Part model, mm, in its own coordinate system. Face numbers are marked on the shaded views. A direction names the side the tool comes from. Coordinates: 2 decimals unless noted, no trailing zeros. Loops run counter-clockwise (first coordinate to the right, second up) from the corner with the lowest first, then second, coordinate; pieces in that order, holes last. Notation, with made-up numbers: (8.5, 51.5) - (44.5, 51.5) arc R14 cw to (44.5, 65.5) - close; hole circle Ø1 at (47.5, -17.5). An arc over 180 degrees is marked (long way). Use a Markdown table: item, result. Add a question column.
1) Pull direction X, two halves, no side cores. Call the marked faces 3 and 4: +X half, -X half, draft (parallel to the pull), parting line (faces both ways), or undercut.
2) Band-saw the part on A-A (x = 23). Give the cut face in (y, z).
3) Band-saw the part on D-D (x = 55). Give the cut face in (y, z), plus the area to 4 significant figures.
4) Drop flat-ended pins along their axis: P1, Ø5.5, axis at x = 23.5, z = 13.5, coming from the -Y side; P2, Ø2, axis at x = 42.5, y = 6, coming from the +Z side; P3, Ø8, axis at y = 44.5, z = 12, coming from the +X side. Give the stop position or say it passes through.
5) Band-saw the part on C-C (y = 95). Give the cut face in (x, z), plus the area to 3 significant figures.
6) Probe probe 1 along X at (y, z) = (143.8, 10.5); probe 2 along Y at (x, z) = (36.5, 8.75); probe 3 along X at (y, z) = (49, 28.75). List the from-to ranges inside material, lowest first. Write a range as [from, to].
7) Tool access for the marked faces 1 and 2: list every direction of +Z, -Z, +X, -X, +Y, -Y with a clear straight run to the whole face (end or side of a thin tool).
8) Band-saw the part on B-B (z = 4.75). Give the cut face in (x, y).
Autodesk Inventor part; units mm, degrees
ref_plane "Work Plane1" through (0, 0, 12.5) normal (0, 0, -1) x (-1, 0, 0)
ref_plane "YZ Plane" through (0, 0, 0) normal (1, 0, 0) x (0, 1, 0)
ref_plane "XZ Plane" through (0, 0, 0) normal (0, 1, 0) x (-1, 0, 0)
sketch "Sketch1" plane through (0, 0, 0) normal (0, 0, 1) x (1, 0, 0)
  line L0 (33.3378, 145.104) -> (83.3378, 145.104)
  line L1 (83.3378, 145.104) -> (83.3378, 5.104)
  line L2 (83.3378, 5.104) -> (33.3378, 5.104)
  line L3 (33.3378, 5.104) -> (33.3378, 145.104)
  line L4 (33.3378, 90.104) -> (33.3378, 60.104)
  line L5 (83.3378, 90.104) -> (83.3378, 60.104)
  point P0 (0, 0)
  dimension "d0" = 140
  dimension "d1" = 50
extrude "Extrusion1" add sketch "Sketch1" along normal blind 30
sketch "Sketch2" plane through (0, 0, 30) normal (0, 0, 1) x (1, 0, 0)
  line L0 (35.8378, 142.604) -> (80.8378, 142.604)
  line L1 (80.8378, 142.604) -> (80.8378, 7.604)
  line L2 (80.8378, 7.604) -> (35.8378, 7.604)
  line L3 (35.8378, 7.604) -> (35.8378, 142.604)
  line L4 (83.3378, 145.104) -> (33.3378, 145.104)
  line L5 (83.3378, 5.104) -> (83.3378, 145.104)
  line L6 (33.3378, 5.104) -> (83.3378, 5.104)
  line L7 (33.3378, 145.104) -> (33.3378, 5.104)
  point P0 (0, 0)
  point P1 (58.3378, 142.604)
  dimension "d4" = 2.5
  dimension "d5" = 2.5
  dimension "d6" = 2.5
  dimension "d7" = 2.5
extrude "Extrusion2" cut sketch "Sketch2" against normal blind 27 contours L0 L1 L2 L3
sketch "Sketch3" plane through (33.3378, 5.104, 0) normal (0, -1, 0) x (1, 0, 0)
  line L0 (7, 30) -> (37, 30)
  line L1 (37, 30) -> (37, 15)
  line L2 (37, 15) -> (7, 15)
  line L3 (7, 15) -> (7, 30)
  line L4 (0, 0) -> (50, 0)
  line L5 (0, 0) -> (0, 30)
  line L6 (0, 30) -> (50, 30)
  line L7 (10, 15) -> (35, 15)
  line L8 (35, 15) -> (35, 3)
  line L9 (35, 3) -> (10, 3)
  line L10 (10, 3) -> (10, 15)
  point P0 (-33.3378, 0)
  point P1 (37, 22.5)
  point P2 (10, 9)
  dimension "d10" = 15
  dimension "d11" = 30
  dimension "d12" = 7
  dimension "d13" = 0
  dimension "d14" = 25
  dimension "d15" = 10
  dimension "d16" = 3
extrude "Extrusion3" cut sketch "Sketch3" against normal blind 27
sketch "Sketch4" plane through (0, 0, 0) normal (0, 0, -1) x (-1, 0, 0)
  circle A0 centre (-74.8378, 13.604) radius 1.5
  circle A1 centre (-41.8378, 13.604) radius 1.5
  circle A2 centre (-41.8378, 99.604) radius 1.5
  circle A3 centre (-74.8378, 99.604) radius 1.5
  circle A4 centre (-41.8378, 111.604) radius 1.5
  circle A5 centre (-74.8378, 111.604) radius 1.5
  line L0 (-83.3378, 5.104) -> (-83.3378, 145.104)
  line L1 (-33.3378, 145.104) -> (-33.3378, 5.104)
  line L2 (-33.3378, 5.104) -> (-83.3378, 5.104)
  line L3 (-83.3378, 145.104) -> (-33.3378, 145.104)
  point P0 (0, 0)
  dimension "d19" = 8.5
  dimension "d20" = 8.5
  dimension "d21" = 8.5
  dimension "d22" = 8.5
  dimension "d23" = 3
  dimension "d24" = 3
  dimension "d25" = 8.5
  dimension "d26" = 8.5
  dimension "d27" = 8.5
  dimension "d28" = 8.5
  dimension "d29" = 3
  dimension "d30" = 3
  dimension "d31" = 3
  dimension "d32" = 3
  dimension "d33" = 12
  dimension "d34" = 12
  dimension "d35" = 33.5
  dimension "d36" = 33.5
extrude "Extrusion4" cut sketch "Sketch4" against normal blind 27 contours A0 | A1 | A2 | A3 | A4 | A5
sketch "Sketch5" plane through (33.3378, 145.104, 0) normal (0, 1, 0) x (1, 0, 0)
  circle A0 centre (35.5, -10.5) radius 2.5
  circle A1 centre (10.5, -10.5) radius 2.5
  line L0 (50, 0) -> (50, -30)
  line L1 (50, 0) -> (0, 0)
  point P0 (-33.3378, 0)
  dimension "d39" = 5
  dimension "d40" = 5
  dimension "d41" = 25
  dimension "d42" = 14.5
  dimension "d43" = 10.5
  dimension "d44" = 10.5
extrude "Extrusion5" cut sketch "Sketch5" against normal blind 27
sketch "Sketch6" plane through (33.3378, 5.104, 0) normal (0, -1, 0) x (1, 0, 0)
  point P0 (-33.3378, 0)
ref_plane "Work Plane1" through (0, 0, 12.5) normal (0, 0, -1) x (-1, 0, 0)
sketch "Sketch7" plane through (0, 0, 12.5) normal (0, 0, -1) x (-1, 0, 0)
  line L0 (-83.3378, 5.104) -> (-83.3378, 145.104)
  line L1 (-83.3378, 90.104) -> (-103.3378, 90.104)
  line L2 (-103.3378, 90.104) -> (-103.3378, 60.104)
  line L3 (-103.3378, 60.104) -> (-83.3378, 60.104)
  line L4 (-83.3378, 60.104) -> (-83.3378, 90.104)
  line L5 (-83.3378, 145.104) -> (-33.3378, 145.104)
  line L6 (-88.3378, 65.104) -> (-98.3378, 65.104)
  line L7 (-98.3378, 65.104) -> (-98.3378, 85.104)
  line L8 (-98.3378, 85.104) -> (-88.3378, 85.104)
  line L9 (-88.3378, 85.104) -> (-88.3378, 65.104)
  line L10 (-33.3378, 145.104) -> (-33.3378, 5.104)
  line L11 (-13.3378, 90.104) -> (-33.3378, 90.104)
  line L12 (-33.3378, 90.104) -> (-33.3378, 60.104)
  line L13 (-33.3378, 60.104) -> (-13.3378, 60.104)
  line L14 (-13.3378, 60.104) -> (-13.3378, 90.104)
  line L15 (-18.3378, 85.104) -> (-28.3378, 85.104)
  line L16 (-28.3378, 85.104) -> (-28.3378, 65.104)
  line L17 (-28.3378, 65.104) -> (-18.3378, 65.104)
  line L18 (-18.3378, 65.104) -> (-18.3378, 85.104)
  point P0 (0, 0)
  point P1 (-93.3378, 60.104)
  dimension "d56" = 20
  dimension "d57" = 30
  dimension "d58" = 55
  dimension "d59" = 5
  dimension "d60" = 20
  dimension "d61" = 30
  dimension "d62" = 55
  dimension "d63" = 5
extrude "Extrusion6" add sketch "Sketch7" along normal mid plane 5
properties part number "arduino mould_3r"
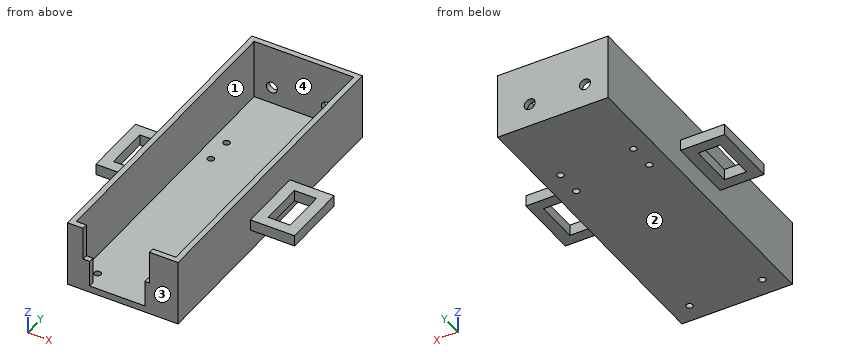
Answer block:
| question | item | result |
|---|---|---|
| 1 | face 3 | draft |
| 1 | face 4 | undercut |
| 2 | outline | (60.1, 10) - (65.1, 10) - (65.1, 15) - (60.1, 15) - close; (85.1, 10) - (90.1, 10) - (90.1, 15) - (85.1, 15) - close |
| 3 | outline | (5.1, 0) - (145.1, 0) - (145.1, 30) - (142.6, 30) - (142.6, 3) - (5.1, 3) - close |
| 3 | area | 487.5 mm2 |
| 4 | P1 | y = 60.1 |
| 4 | P2 | z = 15 |
| 4 | P3 | x = 83.34 |
| 5 | outline | (33.34, 0) - (83.34, 0) - (83.34, 30) - (80.84, 30) - (80.84, 3) - (35.84, 3) - (35.84, 30) - (33.34, 30) - close |
| 5 | area | 285 mm2 |
| 6 | probe 1 | [33.34, 41.34], [46.34, 66.34], [71.34, 83.34] |
| 6 | probe 2 | [5.1, 7.6], [142.6, 145.1] |
| 6 | probe 3 | [33.34, 35.84], [80.84, 83.34] |
| 7 | face 1 | +Z |
| 7 | face 2 | -Z, +X, -X, +Y, -Y |
| 8 | outline | (33.34, 5.1) - (43.34, 5.1) - (43.34, 7.6) - (35.84, 7.6) - (35.84, 142.6) - (80.84, 142.6) - (80.84, 7.6) - (68.34, 7.6) - (68.34, 5.1) - (83.34, 5.1) - (83.34, 145.1) - (33.34, 145.1) - close |
